Check sheet for the drawn part. Datum: minimum x, y, z corner. Units: mm. Coordinates: 2 decimals unless noted, no trailing zeros. Order: outer loops, then holes, each group sorted by start corner. A loop starts at its lowest first (then second) coordinate and runs counter-clockwise, first axis right, second up. Notation, with made-up numbers: (52.25, 7.5) -> (74.25, 7.5) arc R17 cw to (74.25, 26.5) -> close; hole circle Ø4 at (-12, -18). An arc over 180 degrees is marked (long way). Answer as CSV lines item,"result".
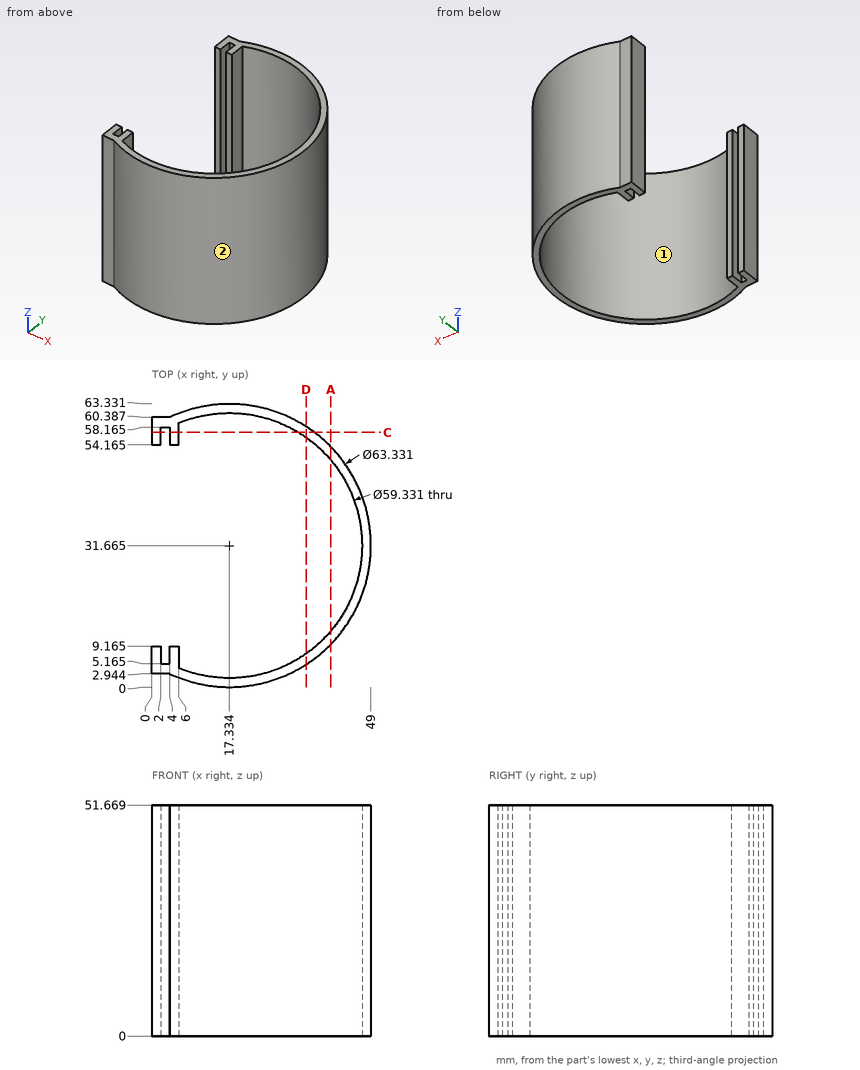
Item 1: Section check C-C, the plane y = 57. Record the boundary of the cut face in (x, z).
Answer list:
outline,"(0, 0) -> (2, 0) -> (2, 51.67) -> (0, 51.67) -> close; (4, 0) -> (6, 0) -> (6, 51.67) -> (4, 51.67) -> close; (32.77, 0) -> (36.33, 0) -> (36.33, 51.67) -> (32.77, 51.67) -> close"
Item 2: Thickness scan on line 1 (X direction, y = 54.5, z = 26.5) (1 decimal); line 2 (Y direction, x = 19, z = 12.5) (1 decimal); line 3 (Y direction, x = 26, z = 47) (1 decimal). Record the ranges inside material, lowest first.
Answer list:
line 1,"0 to 2, 4 to 6, 36.3 to 39.3"
line 2,"0 to 2, 61.3 to 63.3"
line 3,"1.2 to 3.3, 60 to 62.1"
Item 3: Release check for a two-part mould opening along Y. For the marked faces 1 and 2 record: +Y half, -Y half, draft (parallel to the pull), parting line (faces both ways), or undercut.
Answer list:
face 1,"undercut"
face 2,"parting line"
Item 4: Depth check by flat-ended pin: pin 1 Ø1.6 at (x, z) = (1, 27) entering from +Y; pin 2 Ø1 at (x, z) = (13, 23.5) entering from +Y; pin 3 Ø5.5 at (y, z) = (7, 18.5) entering from +X. Enter the tip coordinate at first touch or a pass-through.
Answer list:
pin 1,"y = 60.39"
pin 2,"y = 63.1"
pin 3,"x = 40.19"
Item 5: Section check A-A, the plane x = 40. Record the boundary of the cut face in (y, z) (1 decimal), plus the area to 3 significant figures.
Answer list:
outline,"(9.6, 0) -> (12.5, 0) -> (12.5, 51.7) -> (9.6, 51.7) -> close; (50.8, 0) -> (53.8, 0) -> (53.8, 51.7) -> (50.8, 51.7) -> close"
area,"307 mm2"
Item 6: Section check D-D, the plane x = 34.5. Record the boundary of the cut face in (y, z) (1 decimal).
Answer list:
outline,"(5.1, 0) -> (7.5, 0) -> (7.5, 51.7) -> (5.1, 51.7) -> close; (55.9, 0) -> (58.3, 0) -> (58.3, 51.7) -> (55.9, 51.7) -> close"
